Build history of the part. All positions in model axes, mm. Coordinates: 2 decimals unless noted, no trailing zeros. Order: outer loops, then holes, each group sorted by start corner. A loop starts at its lowest first (then second) coordinate and runs counter-clockwise, first axis right, second up. Notation, with made-up numbers: (72.25, -27.75) - (95.25, -27.75) arc R14 ccw to (95.25, -15.75) - close; hole circle Ø7 at (56.5, 48). An arc over 180 degrees is marked (long way). Write each question's results on one line, items separated by ' | '. Start each with the question number.
Autodesk Inventor part; units mm, degrees
ref_plane "YZ Plane" through (0, 0, 0) normal (1, 0, 0) x (0, 1, 0)
ref_plane "XZ Plane" through (0, 0, 0) normal (0, 1, 0) x (-1, 0, 0)
ref_plane "XY Plane" through (0, 0, 0) normal (0, 0, 1) x (1, 0, 0)
sketch "Sketch1" plane through (0, 0, 0) normal (0, 1, 0) x (-1, 0, 0)
  circle A0 centre (0, 0) radius 177
  dimension "d0" = 354
extrude "Extrusion1" add sketch "Sketch1" along normal blind 4.7625
sketch "Sketch2" plane through (0, 4.7625, 0) normal (0, 1, 0) x (1, 0, 0)
  circle A0 centre (101.6, -101.6) radius 2.1907
  circle A1 centre (101.6, 101.6) radius 2.1907
  circle A2 centre (-101.6, 101.6) radius 2.1907
  circle A3 centre (-101.6, -101.6) radius 2.1907
  circle A4 centre (0, 0) radius 177
  dimension "d3" = 4.3815
  dimension "d4" = 4.3815
  dimension "d5" = 4.3815
  dimension "d6" = 4.3815
  dimension "d14" = 101.6
  dimension "d15" = 101.6
  dimension "d16" = 101.6
  dimension "d17" = 101.6
  dimension "d18" = 101.6
  dimension "d19" = 101.6
  dimension "d20" = 101.6
  dimension "d21" = 101.6
extrude "Standoff Holes" cut sketch "Sketch2" against normal through all contours A0 | A1 | A2 | A3
sketch "Sketch3" plane through (0, 4.7625, 0) normal (0, 1, 0) x (1, 0, 0)
  line L0 (-40, -144.3) -> (40, -144.3)
  line L1 (40, -144.3) -> (40, -114.3)
  line L2 (40, -114.3) -> (-40, -114.3)
  line L3 (-40, -114.3) -> (-40, -144.3)
  circle A0 centre (-25.4, -107.95) radius 1.7
  circle A1 centre (25.4, -107.95) radius 1.7
  circle A2 centre (25.4, -150.65) radius 1.7
  circle A3 centre (-25.4, -150.65) radius 1.7
  circle A4 centre (0, 0) radius 177
  line L4 (-177, 0) -> (177, 0)
  line L5 (-40, 144.3) -> (40, 144.3)
  line L6 (40, 144.3) -> (40, 114.3)
  line L7 (40, 114.3) -> (-40, 114.3)
  line L8 (-40, 114.3) -> (-40, 144.3)
  circle A5 centre (-25.4, 107.95) radius 1.7
  circle A6 centre (25.4, 107.95) radius 1.7
  circle A7 centre (25.4, 150.65) radius 1.7
  circle A8 centre (-25.4, 150.65) radius 1.7
  point P0 (0, -114.3)
  point P1 (0, 114.3)
  dimension "d25" = 80
  dimension "d26" = 30
  dimension "d28" = 114.3
  dimension "d30" = 40
  dimension "d32" = 3.4
  dimension "d33" = 3.4
  dimension "d34" = 3.4
  dimension "d35" = 3.4
  dimension "d36" = 6.35
  dimension "d37" = 6.35
  dimension "d38" = 6.35
  dimension "d39" = 6.35
  dimension "d40" = 25.4
  dimension "d41" = 25.4
  dimension "d42" = 25.4
  dimension "d43" = 25.4
  dimension "d44" = 228.6
extrude "Wheels" cut sketch "Sketch3" against normal blind 25.4 contours L3 L2 L1 L0 | A0 | A1 | A2 | A3 | L5 L6 L7 L8 | A5 | A6 | A7 | A8
sketch "Sketch4" plane through (0, 4.7625, 0) normal (0, 1, 0) x (1, 0, 0)
  circle A0 centre (13.4493, -63.76) radius 1.7
  circle A1 centre (13.4493, -21.9516) radius 1.7
  circle A2 centre (-13.4493, -63.76) radius 1.7
  circle A3 centre (-13.4493, -21.9516) radius 1.7
  line L0 (-40, -114.3) -> (40, -114.3)
  circle A4 centre (0, 0) radius 177
  line L1 (-177, 0) -> (177, 0) construction
  circle A5 centre (13.4493, 63.76) radius 1.7
  circle A6 centre (13.4493, 21.9516) radius 1.7
  circle A7 centre (-13.4493, 63.76) radius 1.7
  circle A8 centre (-13.4493, 21.9516) radius 1.7
  dimension "d47" = 3.4
  dimension "d48" = 3.4
  dimension "d49" = 3.4
  dimension "d50" = 3.4
  dimension "d51" = 26.8986
  dimension "d52" = 26.8986
  dimension "d53" = 41.8084
  dimension "d54" = 41.8084
  dimension "d55" = 13.4493
  dimension "d56" = 13.4493
  dimension "d57" = 50.54
  dimension "d84" = 13.4493
extrude "Motor Mount" cut sketch "Sketch4" against normal through all contours A0 | A1 | A2 | A3 | A5 | A6 | A7 | A8
sketch "Sketch5" plane through (0, 4.7625, 0) normal (0, 1, 0) x (1, 0, 0)
  circle A0 centre (-107.95, -53.7) radius 1.7
  circle A1 centre (-107.95, 38.8) radius 1.7
  circle A2 centre (-29.45, 38.8) radius 1.7
  circle A3 centre (-29.45, -53.7) radius 1.7
  point P0 (0, 0)
  dimension "d61" = 3.4
  dimension "d62" = 3.4
  dimension "d63" = 3.4
  dimension "d64" = 3.4
  dimension "d65" = 92.5
  dimension "d66" = 92.5
  dimension "d67" = 78.5
  dimension "d68" = 78.5
  dimension "d69" = 38.8
  dimension "d70" = 38.8
  dimension "d72" = 53.7
  dimension "d73" = 107.95
extrude "PCB" cut sketch "Sketch5" against normal blind 25.4
sketch "Sketch6" plane through (0, 4.7625, 0) normal (0, 1, 0) x (1, 0, 0)
  circle A0 centre (138.9, -20) radius 1.7
  circle A1 centre (138.9, 20) radius 1.7
  circle A2 centre (0, 0) radius 177
  line L0 (177, 0) -> (177, 59.2823) construction
  line L1 (0, -177) -> (0, 177) construction
  circle A3 centre (-138.9, -20) radius 1.7
  circle A4 centre (-138.9, 20) radius 1.7
  dimension "d76" = 3.4
  dimension "d77" = 3.4
  dimension "d78" = 40
  dimension "d80" = 20
  dimension "d81" = 38.1
extrude "Caster" cut sketch "Sketch6" against normal blind 25.4 contours A0 | A1 | A3 | A4
sketch "Sketch7" plane through (0, 4.7625, 0) normal (0, 1, 0) x (1, 0, 0)
  line L0 (-166.0395, -33.995) -> (-162.8645, -33.995)
  line L1 (-162.8645, -33.995) -> (-162.8645, -27.645)
  line L2 (-162.8645, -27.645) -> (-166.0395, -27.645)
  line L3 (-166.0395, -27.645) -> (-166.0395, -33.995)
  line L4 (-162.8645, -21.295) -> (-162.8645, -14.945)
  line L5 (-162.8645, -14.945) -> (-166.0395, -14.945)
  line L6 (-166.0395, -14.945) -> (-166.0395, -21.295)
  line L7 (-166.0395, -21.295) -> (-162.8645, -21.295)
  line L8 (-162.8645, -8.595) -> (-162.8645, -2.245)
  line L9 (-162.8645, -2.245) -> (-166.0395, -2.245)
  line L10 (-166.0395, -2.245) -> (-166.0395, -8.595)
  line L11 (-166.0395, -8.595) -> (-162.8645, -8.595)
  line L12 (-162.8645, 4.105) -> (-162.8645, 10.455)
  line L13 (-162.8645, 10.455) -> (-166.0395, 10.455)
  line L14 (-166.0395, 10.455) -> (-166.0395, 4.105)
  line L15 (-166.0395, 4.105) -> (-162.8645, 4.105)
  line L16 (-162.8645, 16.805) -> (-162.8645, 23.155)
  line L17 (-162.8645, 23.155) -> (-166.0395, 23.155)
  line L18 (-166.0395, 23.155) -> (-166.0395, 16.805)
  line L19 (-166.0395, 16.805) -> (-162.8645, 16.805)
  line L20 (-162.8645, 29.505) -> (-162.8645, 35.855)
  line L21 (-162.8645, 35.855) -> (-166.0395, 35.855)
  line L22 (-166.0395, 35.855) -> (-166.0395, 29.505)
  line L23 (-166.0395, 29.505) -> (-162.8645, 29.505)
  point P0 (0, 0)
  dimension "d85" = 6.35
  dimension "d86" = 3.175
  dimension "d89" = 12.7
  dimension "d94" = 162.8645
  dimension "d95" = 33.995
extrude "Switch" cut sketch "Sketch7" against normal through all
sketch "Sketch8" plane through (0, 4.7625, 0) normal (0, 1, 0) x (1, 0, 0)
  circle A0 centre (121.3, 5.9) radius 1.7
  circle A1 centre (114.3, -5.9) radius 1.7
  point P0 (0, 0)
  dimension "d98" = 3.4
  dimension "d99" = 3.4
  dimension "d100" = 11.8
  dimension "d101" = 7
  dimension "d102" = 5.9
  dimension "d103" = 114.3
extrude "Extrusion8" cut sketch "Sketch8" against normal blind 25.4
equation "\"d3\" = d4"
equation "\"d5\" = d4"
equation "\"d6\" = d4"
equation "\"d52\" = d51"
equation "\"d54\" = d53"
equation "\"d62\" = d61"
equation "\"d63\" = d61"
equation "\"d64\" = d61"
equation "\"d66\" = d65"
equation "\"d68\" = d67"
equation "\"d98\" = m3_clearance"
equation "\"d99\" = m3_clearance"
equation "\"m3_heat_set_insert\" = 4"
equation "\"m3_clearance\" = 3.4"
equation "\"m3_heat_set_depth\" = 7"
equation "\"robot_diameter\" = 354"
equation "\"hardboard_thickness\" = 5"
equation "\"motor_centerline_height\" = 13"
properties part number "layer1"
Item 1: Slice it at B-B (y = 1.4). Count the separate pieces of the cut face and the enclosed holes in it, then the cut area to 3 significant figures.
Item 2: Slice it at A-A (x = -6). Write the cut outline in (y, z), then the cut area to 3 significant figures.
Item 3: Slice it at D-D (z = -49). Write the cut outline in (x, y), then the cut area to 3 significant figures.
Item 4: Probe probe 1 along X at (y, z) = (2.6, 150.65); probe 2 along X at (y, z) = (2.35, -107.95); probe 3 along Z at (x, y) = (-17, 0.3). List the from-to ranges inside material, lowest first.
Item 5: Slice it at C-C (x = 86). Write the cut outline in (y, z), then the cut area to 3 significant figures.
Item 6: Flat gauge pins, fed straight in: P1, Ø2, axis at y = 4, z = -30.5, coming from the -X side; P2, Ø2.5, axis at x = -164.5, y = 3.5, coming from the +Z side; P3, Ø1, axis at x = -108.5, y = 1.5, coming from the -Z side. Where does each tip first touch, or does it go through?
Resolved:
1) separate pieces: 1 | enclosed holes: 38 | area: 93,200 mm^2
2) outline: (0, -176.9) - (4.76, -176.9) - (4.76, -144.3) - (0, -144.3) - close; (0, -114.3) - (4.76, -114.3) - (4.76, 114.3) - (0, 114.3) - close; (0, 144.3) - (4.76, 144.3) - (4.76, 176.9) - (0, 176.9) - close | area: 1,400 mm^2
3) outline: (-170.08, 0) - (170.08, 0) - (170.08, 4.76) - (-170.08, 4.76) - close | area: 1,620 mm^2
4) probe 1: -92.92 to -27.1, -23.7 to 23.7, 27.1 to 92.92 | probe 2: -140.27 to -27.1, -23.7 to 23.7, 27.1 to 140.27 | probe 3: -176.18 to -144.3, -114.3 to 114.3, 144.3 to 176.18
5) outline: (0, -154.7) - (4.76, -154.7) - (4.76, 154.7) - (0, 154.7) - close | area: 1,470 mm^2
6) P1: x = -174.52 | P2: z = 68.4 | P3: z = -140.23
